For this review, take the finished solid that the model builds, in its own axes (mm). Face numbers are marked on the shaded views. A direction names the side the tool comes from. Round coordinates to 2 decimals unless told otherwise and drop trailing zeros. Write each loop counter-clockwise with the first axis right and the second up, starting at its lowest first coordinate (ties: lowest second). Pieces come first, ordered by that corner, then holes. Notation, with made-up numbers: (-23, 39.25) -> (7, 39.25) arc R27 cw to (7, 67.25) -> close; hole circle Ø8 at (84.5, 64.5). An arc over 180 degrees is marked (long way). Answer in a Markdown table with one row per item. Add a question column.
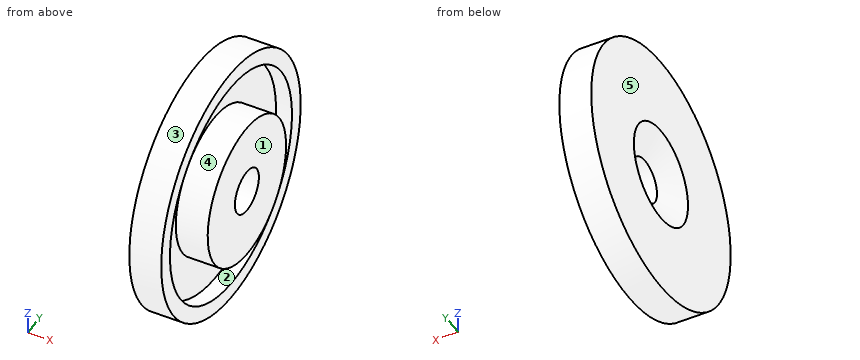
```python
from build123d import *

# Parameters (mm, degrees)
SKETCH_1_R      = 14
SKETCH_1_R_2    = 9
EXTRUDE_1_DEPTH = 2
SKETCH_1_3_R    = 16
SKETCH_1_3_R_2  = 14
EXTRUDE_2_DEPTH = 4
SKETCH_1_4_R    = 9
SKETCH_1_4_R_2  = 2.75
EXTRUDE_3_DEPTH = 6
CHAMFER_1_SIZE  = 2
CHAMFER_1_SIZE2 = 3.464101615


with BuildPart() as part:
    # 草图1 → 凸台-拉伸1 (new body)
    with BuildSketch(Plane(origin=(0, 0, 0), x_dir=(0, 0, -1), z_dir=(1, 0, 0))):
        Circle(SKETCH_1_R)
        Circle(SKETCH_1_R_2, mode=Mode.SUBTRACT)
    extrude(amount=EXTRUDE_1_DEPTH)

    # 草图1<3> → 凸台-拉伸2 (add)
    with BuildSketch(Plane(origin=(0, 0, 0), x_dir=(0, 0, -1), z_dir=(1, 0, 0))):
        Circle(SKETCH_1_3_R)
        Circle(SKETCH_1_3_R_2, mode=Mode.SUBTRACT)
    extrude(amount=EXTRUDE_2_DEPTH)

    # 草图1<4> → 凸台-拉伸3 (add)
    with BuildSketch(Plane(origin=(0, 0, 0), x_dir=(0, 0, -1), z_dir=(1, 0, 0))):
        Circle(SKETCH_1_4_R)
        Circle(SKETCH_1_4_R_2, mode=Mode.SUBTRACT)
    extrude(amount=EXTRUDE_3_DEPTH)

    # 倒角1
    chamfer_1_edges = [part.edges().sort_by_distance(p)[0] for p in [
        (0, 0, 2.75),
    ]]
    chamfer_1_side = [part.faces().sort_by_distance(p)[0] for p in [
        (3, 0, 2.75),
    ]]
    chamfer(chamfer_1_edges, length=CHAMFER_1_SIZE, length2=CHAMFER_1_SIZE2, reference=chamfer_1_side[0])


solid = part.part
```
1. We need section A-A (y = 0). Write out the cut boundary in (x, z).
2. Clearance check with flat-ended pins moving along their axes: pin 1 Ø3 at (x, z) = (3, -5) entering from +Y; pin 2 Ø6.5 at (y, z) = (0, 0) entering from -X; pin 3 Ø1.5 at (x, z) = (0.5, -4.5) entering from -Y. State where each tip first meets the part, or that it passes through.
3. The part is to be moulded in two halves that separate along Y. For the marked faces 1, 2 and 3, say which applies: pulls with the +Y half, pulls with the -Y half, needs draft (parallel to the pull), parting line crosses it, or undercut.
4. Tool access review of the marked faces 4 and 5: name each direction out of +Z, -Z, +X, -X, +Y, -Y from which nothing blocks a thin tool from reaching the whole face with its end or side.
5. We need section D-D (x = 4.9). Write out the cut boundary in (y, z), plus the area to 3 significant figures.
6. For L1, parallel to Y at x = 3.65, z = 0; L2, parallel to Y at x = 4.75, z = 0; L3, parallel to X at y = -9.5, z = 0.5, list the stretches that pass through material, from the lowest coordinate up. Write a range as [from, to].
7. We need section C-C (x = 2.9). Write out the cut boundary in (y, z).
Response:
| question | item | result |
|---|---|---|
| 1 | outline | (0, -16) -> (4, -16) -> (4, -14) -> (2, -14) -> (2, -9) -> (6, -9) -> (6, -2.75) -> (2, -2.75) -> (0, -6.21) -> close; (0, 6.21) -> (2, 2.75) -> (6, 2.75) -> (6, 9) -> (2, 9) -> (2, 14) -> (4, 14) -> (4, 16) -> (0, 16) -> close |
| 2 | pin 1 | y = 15.61 |
| 2 | pin 2 | x = 1.71 |
| 2 | pin 3 | y = -15.55 |
| 3 | face 1 | needs draft |
| 3 | face 2 | undercut |
| 3 | face 3 | parting line crosses it |
| 4 | face 4 | +X |
| 4 | face 5 | +Z, -Z, -X, +Y, -Y |
| 5 | outline | circle Ø18 at (0, 0); hole circle Ø5.5 at (0, 0) |
| 5 | area | 231 mm2 |
| 6 | L1 | [-16, -14], [-9, -2.75], [2.75, 9], [14, 16] |
| 6 | L2 | [-9, -2.75], [2.75, 9] |
| 6 | L3 | [0, 2] |
| 7 | outline | circle Ø32 at (0, 0); circle Ø18 at (0, 0); hole circle Ø28 at (0, 0); hole circle Ø5.5 at (0, 0) |
